Work out the finished part from the listing and answer in its coordinate system (mm). A direction names the side the tool comes from. Coordinates: 2 decimals unless noted, no trailing zeros. Answer as CSV lines item,"result". Start each with the question number.
(1) The mould has two halves that part along Z. Classify faces 5 (the flat face through (-10.5, -10, 7)), 6 (the cylindrical face through (-9.76, -3.604, 11.446)), 7 (the cylindrical face through (-6.226, -6.324, 4.032)): released by +Z, released by -Z, zero draft, split by the parting line, or undercut.
(2) For faces 1 (the flat face through (0, 0, -9)), 2 (the cylindrical face through (-9.7, -3.2, 10)), 3 (the flat face through (-1.5, -9, 0)), 4 (the cylindrical face through (-0.74, -8.428, -1.107)), determine the directions among +Z, -Z, +X, -X, +Y, -Y from which every point of the face is accessible in a straight line to the end or side of a thin tool.
(3) Flat-ended cylindrical pins translate along their axes: P1, Ø9, axis at y = -0.5, z = -3, coming from the -X side; P2, Ø3, axis at x = -3.5, y = 4, coming from the +Z side; P3, Ø6, axis at x = -5.5, y = 6.5, coming from the +Z side. Find the tip coordinate at first contact, or state that the pin passes through.
(4) Find the intervals of material crossed by L1, parallel to Y at x = -9.75, z = 0; L2, parallel to X at y = 5, z = -7.25; L3, parallel to Y at x = -0.8, z = 0, in increasing order. Write a range as [from, to].
from build123d import *

# Parameters (mm, degrees)
CONG_1_R = 0.5


with BuildPart() as part:
    # Esquisse1 → Révolution1 (revolve)
    with BuildSketch(Plane.XY, mode=Mode.PRIVATE) as r_volution1_sk:
        Polygon((-8, 7.5), (-4.5, 7.5), (-4.5, 9.815), (-1.5, 9.815), (-1.5, 8.5), (0, 8.5), (0, 10.5), (-9, 15), (-9, 12), (-10.5, 12), (-10.5, 12.5), (-11.5, 12.5), (-11.5, 10.5), (-8, 10.5), align=None)
    revolve(r_volution1_sk.sketch.rotate(Axis((-27.606261023, 0, 0), (1, 0, 0)), 90), axis=Axis((-27.606261023, 0, 0), (1, 0, 0)))  # turned: the seam where the file's is

    # Congé1
    cong_1_edges = [part.edges().sort_by_distance(p)[0] for p in [
        (-11.5, 0, -12.5),
    ]]
    fillet(cong_1_edges, radius=CONG_1_R)


solid = part.part
Here are the results:
1,face 5,"zero draft"
1,face 6,"split by the parting line"
1,face 7,"undercut"
2,face 1,"+Z, -Z, +X, +Y, -Y"
2,face 2,"-X"
2,face 3,"none"
2,face 4,"+X"
3,P1,"stops at x = -8"
3,P2,"stops at z = 12.48"
3,P3,"stops at z = 13.67"
4,L1,"y = [-12, -10.5], [10.5, 12]"
4,L2,"x = [-8, -4.5], [-1.5, 0]"
4,L3,"y = [-10.9, -8.5], [8.5, 10.9]"
